```python
from build123d import *

# Parameters (mm, degrees)
F2_W      = 5
F2_H      = 120
F3_DEPTH  = 30
F0_W      = 180
F0_H      = 140
F4_DEPTH  = 10
F5_W      = 5
F5_H      = 120
F6_DEPTH  = 25
F9_W      = 5
F9_H      = 120
F10_DEPTH = 27.9
F12_W     = 5
F12_H     = 120
F13_DEPTH = 33.6
F14_W     = 5
F14_H     = 120
F15_DEPTH = 27.3
F17_W     = 5
F17_H     = 120
F18_DEPTH = 32
F19_W     = 5
F19_H     = 120
F20_DEPTH = 25.9
F22_W     = 10
F22_H     = 10
F23_DEPTH = 13
F26_DEPTH = 15


with BuildPart() as f3:
    # F2 (on line) → F3 (new body)
    with BuildSketch(Plane(origin=(-8.5942352531, 0, 26.4503363532), x_dir=(0.9510565163, 0, 0.3090169944), z_dir=(0.3090169944, 0, -0.9510565163))):
        with Locations((-73.0950864666, 0.9517986327)):
            Rectangle(F2_W, F2_H)
    extrude(amount=-F3_DEPTH)

    # F0 (on Top) → F4 (join)
    with BuildSketch(Plane.XY):
        Rectangle(F0_W, F0_H)
    extrude(amount=F4_DEPTH)

    # F5 (on line) → F6 (join)
    with BuildSketch(Plane(origin=(-8.5942352531, 0, 26.4503363532), x_dir=(0.9510565163, 0, 0.3090169944), z_dir=(0.3090169944, 0, -0.9510565163))):
        with Locations((-53.0950864666, 0)):
            Rectangle(F5_W, F5_H)
    extrude(amount=-F6_DEPTH)

    # F9 (on line) → F10 (join)
    with BuildSketch(Plane(origin=(-5.7232027477, 0, 17.6142068765), x_dir=(0.9510565163, 0, 0.3090169944), z_dir=(0.3090169944, 0, -0.9510565163))):
        with Locations((-33.0950864666, 0)):
            Rectangle(F9_W, F9_H)
    extrude(amount=-F10_DEPTH)

    # F12 (on line) → F13 (join)
    with BuildSketch(Plane(origin=(-2.029499084, 0, 6.2461559196), x_dir=(0.9510565163, 0, 0.3090169944), z_dir=(0.3090169944, 0, -0.9510565163))):
        with Locations((-13.0950864666, 0)):
            Rectangle(F12_W, F12_H)
    extrude(amount=-F13_DEPTH)

    # F14 (on line) → F15 (join)
    with BuildSketch(Plane(origin=(-2.029499084, 0, 6.2461559196), x_dir=(0.9510565163, 0, 0.3090169944), z_dir=(0.3090169944, 0, -0.9510565163))):
        with Locations((6.9049135334, 0)):
            Rectangle(F14_W, F14_H)
    extrude(amount=-F15_DEPTH)

    # F17 (on line) → F18 (join)
    with BuildSketch(Plane(origin=(1.5478064215, 0, -4.7636583421), x_dir=(0.9510565163, 0, 0.3090169944), z_dir=(0.3090169944, 0, -0.9510565163))):
        with Locations((26.9049135334, 0)):
            Rectangle(F17_W, F17_H)
    extrude(amount=-F18_DEPTH)

    # F19 (on line) → F20 (join)
    with BuildSketch(Plane(origin=(1.5478064215, 0, -4.7636583421), x_dir=(0.9510565163, 0, 0.3090169944), z_dir=(0.3090169944, 0, -0.9510565163))):
        with Locations((46.9049135334, 0)):
            Rectangle(F19_W, F19_H)
    extrude(amount=-F20_DEPTH)

    # F22 (on offset) → F23 (join)
    with BuildSketch(Plane.XY.offset(10)):
        with Locations((62.2089297195, 34.1514503138)):
            Rectangle(F22_W, F22_H)
        with Locations((62.2089297195, -13.2830284653)):
            Rectangle(F22_W, F22_H)
    extrude(amount=F23_DEPTH)

    # F25 (on face) + F24 (on face) → F26 (cut)
    with BuildSketch(Plane.YZ.offset(67.2089297195)):
        Polygon((-13.2830284653, 20), (-18.2830284653, 23), (-18.2830284653, 10), (-13.2830284653, 10), align=None)
    with BuildSketch(Plane.YZ.offset(67.2089297195)):
        Polygon((39.1514503138, 10), (39.1514503138, 23), (34.1514503138, 20), (34.1514503138, 10), align=None)
    extrude(amount=-F26_DEPTH, mode=Mode.SUBTRACT)


solid = f3.part
```
Input: part model. Units: mm. Frame: model coordinates. A direction names the side the tool comes from. Coordinates: 2 decimals unless noted, no trailing zeros. Loops run counter-clockwise (first coordinate to the right, second up) from the corner with the lowest first, then second, coordinate; pieces in that order, holes last. Notation, with made-up numbers: (-18.5, 66.25) - (14.5, 66.25) arc R18 cw to (14.5, 76.25) - close; hole circle Ø8 at (-24.5, 27.25). An arc over 180 degrees is marked (long way). Answer in a Markdown table with one row per item.
(1) Cut plane C-C on x = -4. Output: boundary loops of the cut face in (y, z), plus the area to 3 significant figures.
Model answer:
| item | result |
|---|---|
| outline | (-70, 0) - (70, 0) - (70, 10) - (-70, 10) - close; (-60, 26.57) - (60, 26.57) - (60, 34.31) - (-60, 34.31) - close |
| area | 2,330 mm² |
(2) Material intervals for L1, parallel to Y at x = -21, z = 25; L2, parallel to Z at x = -35, y = 51, sorted ascending. Write a range as from..to.
Model answer:
| item | result |
|---|---|
| L1 | y = -60..60 |
| L2 | z = 0..10 |
(3) Mould query, pull axis X, two halves, no side actions, for faces 1 (the face through (-90, -1, 5)), 2 (the face through (-23.392, 0.84, 21.528)), 3 (the face through (-63, -60, 22)). Classes: pulls with the +X half, pulls with the -X half, needs draft (parallel to the pull), parting line crosses it, or undercut.
Model answer:
| item | result |
|---|---|
| face 1 | pulls with the -X half |
| face 2 | undercut |
| face 3 | needs draft |
(4) Pin query (flat end, axial travel): P1, Ø3, axis at y = -13, z = 16, coming from the -X side; P2, Ø10.5, axis at x = 2, z = 25.5, coming from the -Y side; P3, Ø3, axis at x = 64, y = -13, coming from the +Z side. Return the tip coordinate at first contact, or that it passes through.
Model answer:
| item | result |
|---|---|
| P1 | stops at x = -85.17 |
| P2 | stops at y = -60 |
| P3 | stops at z = 23 |
(5) Cut plane D-D on x = 53. Output: boundary loops of the cut face in (y, z), plus the area to 3 significant figures.
Model answer:
| item | result |
|---|---|
| outline | (-70, 0) - (70, 0) - (70, 10) - (-70, 10) - close |
| area | 1,400 mm² |
(6) Cut plane A-A on z = 28. Output: boundary loops of the cut face in (x, y), plus the area to 3 significant figures.
Model answer:
| item | result |
|---|---|
| outline | (-88.58, -60.95) - (-83.33, -60.95) - (-83.33, 59.05) - (-88.58, 59.05) - close; (-67.55, -60) - (-62.3, -60) - (-62.3, 60) - (-67.55, 60) - close; (-46.52, -60) - (-41.27, -60) - (-41.27, 60) - (-46.52, 60) - close; (-25.5, -60) - (-20.24, -60) - (-20.24, 60) - (-25.5, 60) - close; (-4.47, -60) - (0.79, -60) - (0.79, 60) - (-4.47, 60) - close; (16.56, -60) - (21.82, -60) - (21.82, 60) - (16.56, 60) - close; (37.59, -60) - (42.85, -60) - (42.85, 60) - (37.59, 60) - close |
| area | 4,420 mm² |
(7) Set-up query: faces 4 (the face through (62.28, -15.75, 21.48)), 5 (the face through (57.209, 32, 16)), 6 (the face through (21, -60, 21)). Return all of +Z, -Z, +X, -X, +Y, -Y with unobstructed straight access to the full face (end or side cutting, diameter ignored); none if empty.
Model answer:
| item | result |
|---|---|
| face 4 | +X, -Y |
| face 5 | +Z, +Y, -Y |
| face 6 | +Z, +X, -Y |
